Could you check a few things on this drawing? It's one solid part, dimensions in mm from its lowest x, y, z. A direction names the side the tool comes from. Give positions to 0.01 mm unless a question says otherwise; leave off trailing zeros. Loops run counter-clockwise (first coordinate to the right, second up) from the corner with the lowest first, then second, coordinate; pieces in that order, holes last.
Q1. I need wall thicknesses on probe 1 along Z at (x, y) = (5, 3); probe 2 along Y at (x, z) = (12, 9); probe 3 along Y at (x, z) = (3.5, 29). Which ranges of each line are inside material? Lowest first, please.
Q2. I'm going to push flat-ended pins straight in: P1, Ø3, axis at y = 6, z = 5.5, coming from the -X side; P2, Ø5, axis at y = 17, z = 15, coming from the +X side; P3, Ø8, axis at y = 8, z = 10.5, coming from the +X side. Where does each tip first touch, or does it pass through?
Q3. Suppose I cut it at D-D (z = 3.5). List the corners of the cut face in (x, y) for me, and give its area (3 significant figures).
Q4. Suppose I cut it at B-B (y = 1.5). List the corners of the cut face in (x, z) for me, and give its area (3 significant figures).
Q5. For the marked faces 1 and 2, which set-ups out of +Z, -Z, +X, -X, +Y, -Y let a thin tool reach every point of the face, with its end or its side?
Q6. Suppose I cut it at A-A (x = 10). List the corners of the cut face in (y, z) for me, and give its area (3 significant figures).
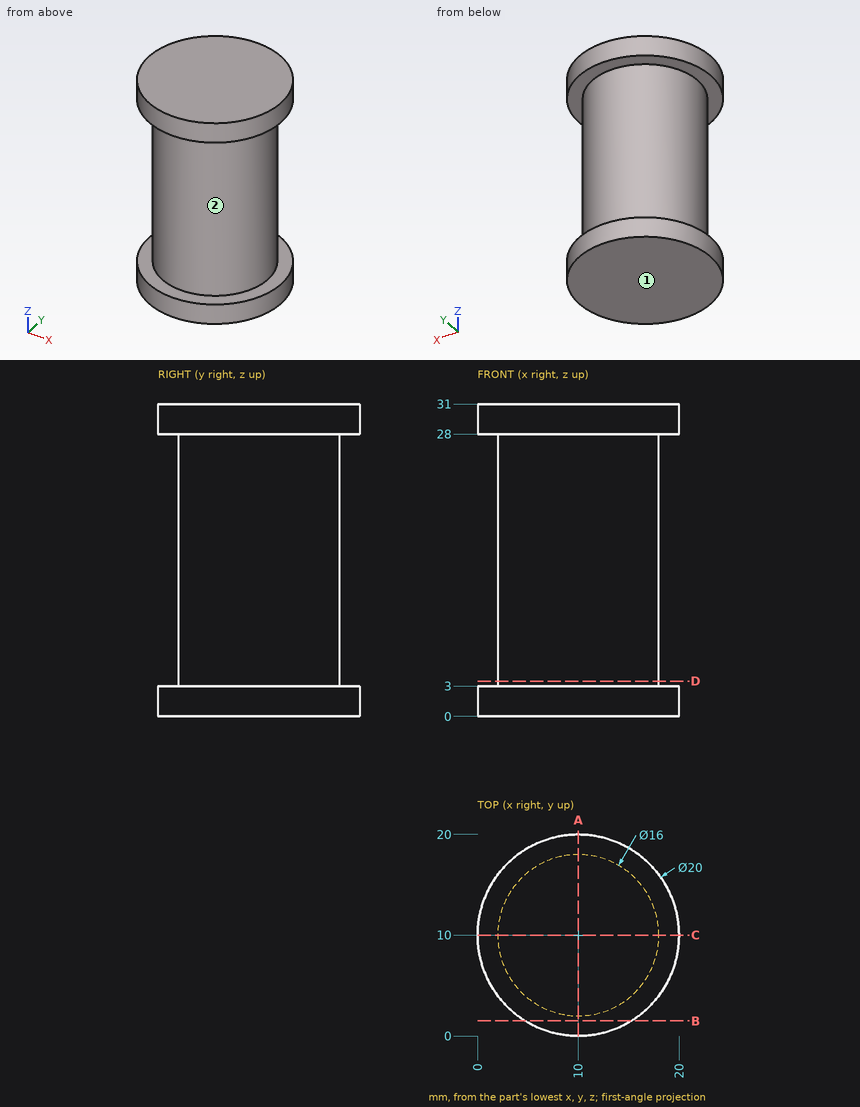
Solutions:
1. probe 1: z = 0 to 3, 28 to 31
1. probe 2: y = 2.25 to 17.75
1. probe 3: y = 2.4 to 17.6
2. P1: stops at x = 2.4
2. P2: stops at x = 16.61
2. P3: stops at x = 18
3. outline: circle Ø16 at (10, 10)
3. area: 201 mm2
4. outline: (4.73, 0) - (15.27, 0) - (15.27, 3) - (4.73, 3) - close; (4.73, 28) - (15.27, 28) - (15.27, 31) - (4.73, 31) - close
4. area: 63.2 mm2
5. face 1: -Z, +X, -X, +Y, -Y
5. face 2: none
6. outline: (0, 0) - (20, 0) - (20, 3) - (18, 3) - (18, 28) - (20, 28) - (20, 31) - (0, 31) - (0, 28) - (2, 28) - (2, 3) - (0, 3) - close
6. area: 520 mm2
